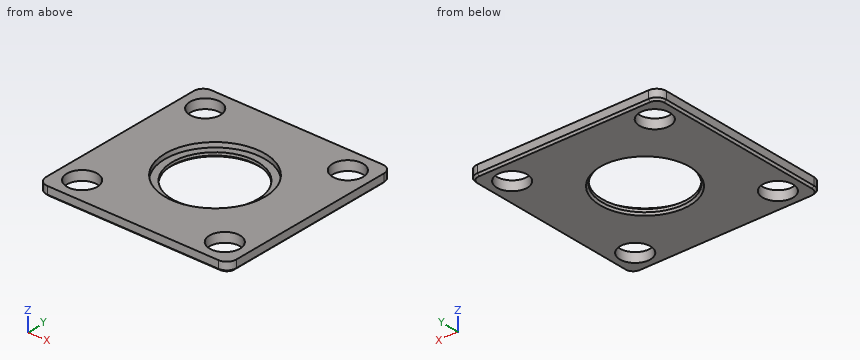
Autodesk Inventor part; units mm, degrees
ref_plane "YZ Plane" through (0, 0, 0) normal (1, 0, 0) x (0, 1, 0)
ref_plane "XZ Plane" through (0, 0, 0) normal (0, 1, 0) x (-1, 0, 0)
ref_plane "XY Plane" through (0, 0, 0) normal (0, 0, 1) x (1, 0, 0)
sketch "Sketch1" plane through (0, 0, 0) normal (0, 0, 1) x (1, 0, 0)
  line L0 (-20, 20) -> (20, 20)
  line L1 (20, 20) -> (20, -20)
  line L2 (20, -20) -> (-20, -20)
  line L3 (-20, -20) -> (-20, 20)
  point P0 (0, 0)
  point P1 (20, 0)
  point P2 (0, 20)
  dimension "d0" = 40
extrude "Extrusion1" add sketch "Sketch1" along normal blind 2
fillet "Fillet1" radius 2 4 edges at (20, 20, 1) (-20, 20, 1) (20, -20, 1) (-20, -20, 1)
sketch "Sketch2" plane through (0, 0, 2) normal (0, 0, 1) x (1, 0, 0)
  line L0 (-15, 15) -> (15, 15) construction
  line L1 (15, 15) -> (15, -15) construction
  line L2 (15, -15) -> (-15, -15) construction
  line L3 (-15, -15) -> (-15, 15) construction
  point P0 (0, 0)
  point P1 (15, 0)
  point P2 (0, 15)
  dimension "d4" = 30
hole "Hole1" at (-15, 15, 2) at (15, 15, 2) at (15, -15, 2) at (-15, -15, 2) direction (0, 0, -1) diameter 6.4 end through all
sketch "Sketch3" plane through (0, 0, 2) normal (0, 0, 1) x (1, 0, 0)
  circle A0 centre (0, 0) radius 10.5
  dimension "d12" = 21
extrude "Extrusion2" cut sketch "Sketch3" against normal blind 1
sketch "Sketch4" plane through (0, 0, 1) normal (0, 0, 1) x (1, 0, 0)
  circle A0 centre (0, 0) radius 9
  dimension "d15" = 18
extrude "Extrusion3" cut sketch "Sketch4" against normal through all
chamfer "Chamfer1" distance 0.4 angle 45 9 edges at (-9, 0, 0) (0, -20, 0) (19.4142, -19.4142, 0) (20, 0, 0) (19.4142, 19.4142, 0) (0, 20, 0) (-19.4142, 19.4142, 0) (-20, 0, 0) (-19.4142, -19.4142, 0)
properties part number "RamanSampleHolder"
Geometry: final body of the model. Coordinates: model frame, mm. Round coordinates to 2 decimals unless told otherwise and drop trailing zeros. Write each loop counter-clockwise with the first axis right and the second up, starting at its lowest first coordinate (ties: lowest second). Pieces come first, ordered by that corner, then holes.
Item 1: Section query B-B (z = 1.45). Return loops of the section in (x, y), plus the area to 3 significant figures.
Item 2: Section query A-A (y = 0). Return loops of the section in (x, z), plus the area to 3 significant figures.
Item 3: Section query C-C (y = 15). Return loops of the section in (x, z).
Item 4: Material intervals for L1, parallel to X at y = -15, z = 0.6; L2, parallel to Y at x = 17.5, z = 1.6, sorted ascending.
Completed:
1. outline: (-20, -18) arc R2 ccw to (-18, -20) - (18, -20) arc R2 ccw to (20, -18) - (20, 18) arc R2 ccw to (18, 20) - (-18, 20) arc R2 ccw to (-20, 18) - close; hole circle Ø6.4 at (-15, -15); hole circle Ø6.4 at (-15, 15); hole circle Ø21 at (0, 0); hole circle Ø6.4 at (15, -15); hole circle Ø6.4 at (15, 15)
1. area: 1,120 mm2
2. outline: (-20, 0.4) - (-19.6, 0) - (-9.4, 0) - (-9, 0.4) - (-9, 1) - (-10.5, 1) - (-10.5, 2) - (-20, 2) - close; (9, 0.4) - (9.4, 0) - (19.6, 0) - (20, 0.4) - (20, 2) - (10.5, 2) - (10.5, 1) - (9, 1) - close
2. area: 40.7 mm2
3. outline: (-20, 0.4) - (-19.6, 0) - (-18.2, 0) - (-18.2, 2) - (-20, 2) - close; (-11.8, 0) - (11.8, 0) - (11.8, 2) - (-11.8, 2) - close; (18.2, 0) - (19.6, 0) - (20, 0.4) - (20, 2) - (18.2, 2) - close
4. L1: x = -20 to -18.2, -11.8 to 11.8, 18.2 to 20
4. L2: y = -20 to -17, -13 to 13, 17 to 20
